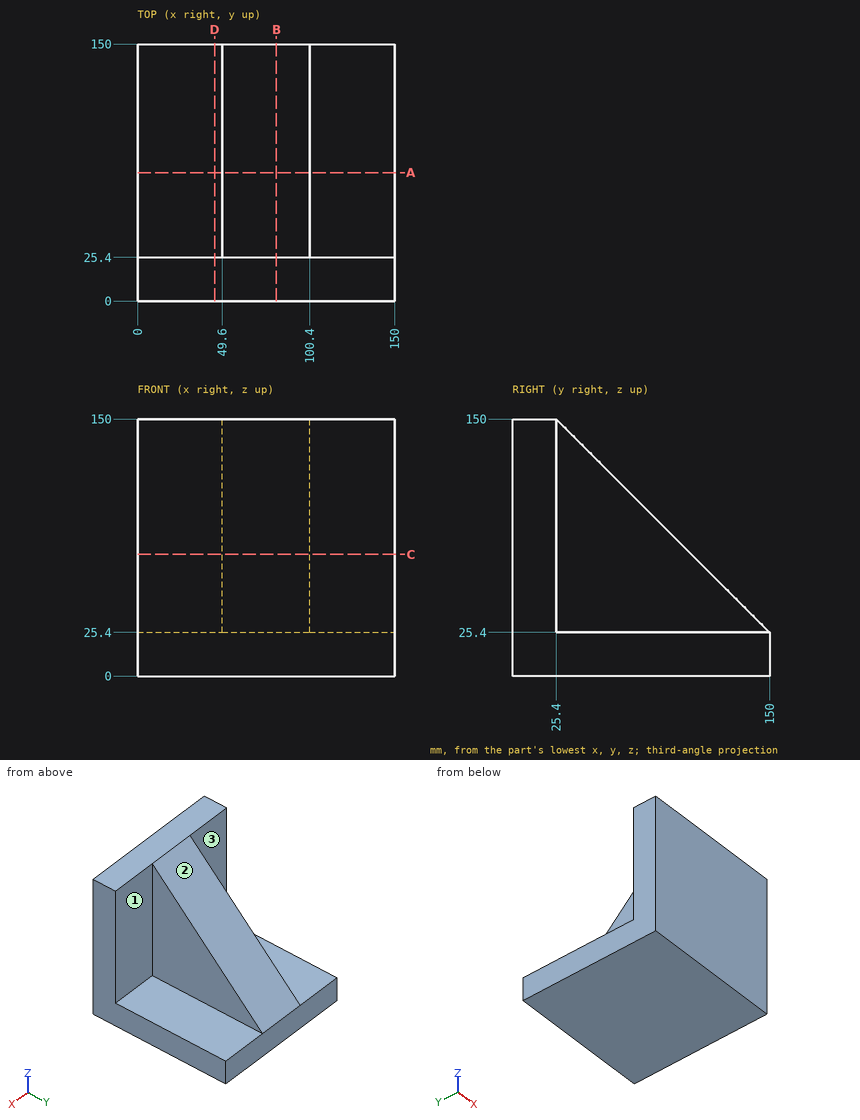
For this review, use the dimensioned drawing (mm, ordinates from the lowest corner) and the shaded views. A direction names the side the tool comes from. Give positions to 0.01 mm unless a question says otherwise; leave off trailing zeros. Write each loop counter-clockwise with the first axis right and the second up, starting at its lowest first coordinate (ties: lowest second). Pieces come first, ordered by that corner, then holes.
(1) To check wall thickness, follow L1, parallel to Y at x = 113.5, z = 127; L2, parallel to X at y = 64.5, z = 47.5. State the ranges of each line that lie inside material, in increasing order.
(2) Tool access review of the marked faces 1, 2 and 3: name each direction out of +Z, -Z, +X, -X, +Y, -Y from which nothing blocks a thin tool from reaching the whole face with its end or side.
(3) Consider section C-C, the plane z = 71. Give the boundary of the cut face in (x, y).
(4) Consider section D-D, the plane x = 45. Give the boundary of the cut face in (y, z).
(5) Consider section A-A, the plane y = 75. Give the boundary of the cut face in (x, z).
(6) Consider section B-B, the plane x = 81. Give the boundary of the cut face in (y, z), and give its area (3 significant figures).
(7) For P1, Ø2, axis at x = 112.5, z = 70.5, coming from the +Y side; P2, Ø8, axis at x = 93, y = 103.5, coming from the +Z side; P3, Ø25, axis at x = 16.5, y = 105, coming from the +Z side, all flat-tipped, find the tip position at first contact; note any pin that passes through.
Returned:
1. L1: y = 0 to 25.4
1. L2: x = 49.6 to 100.4
2. face 1: +Z, +X, +Y
2. face 2: +Z, +X, -X, +Y
2. face 3: +Z, -X, +Y
3. outline: (0, 0) - (150, 0) - (150, 25.4) - (100.4, 25.4) - (100.4, 104.4) - (49.6, 104.4) - (49.6, 25.4) - (0, 25.4) - close
4. outline: (0, 0) - (150, 0) - (150, 25.4) - (25.4, 25.4) - (25.4, 150) - (0, 150) - close
5. outline: (0, 0) - (150, 0) - (150, 25.4) - (100.4, 25.4) - (100.4, 100.4) - (49.6, 100.4) - (49.6, 25.4) - (0, 25.4) - close
6. outline: (0, 0) - (150, 0) - (150, 25.4) - (25.4, 150) - (0, 150) - close
6. area: 14,700 mm2
7. P1: stops at y = 25.4
7. P2: stops at z = 75.9
7. P3: stops at z = 25.4
